The model under review builds one solid part; all positions refer to its coordinate system, in mm. Face numbers are marked on the shaded views. A direction names the side the tool comes from. Round coordinates to 2 decimals unless told otherwise and drop trailing zeros. Loops run counter-clockwise (first coordinate to the right, second up) from the corner with the lowest first, then second, coordinate; pieces in that order, holes last. Notation, with made-up numbers: (77, -7.5) -> (117, -7.5) arc R26 ccw to (117, 9.5) -> close; hole circle Ø3 at (21, 16.5). An arc over 180 degrees is marked (long way). Use CSV: the item, a comma, the result in double quotes. Start each with the question number.
```python
from build123d import *

# Parameters (mm, degrees)
SKETCH1_R               = 27.274244274
SKETCH1_R_2             = 12.5
BOSS_EXTRUDE1_DEPTH     = 2
SKETCH4_R               = 15
BOSS_EXTRUDE3_DEPTH     = 7
SKETCH5_R               = 6
SKETCH5_R_2             = 4.1
BOSS_EXTRUDE4_DEPTH     = 10
CUT_EXTRUDE1_DEPTH      = 43.997311561
CUT_EXTRUDE1_DEPTH_BACK = 43.997311561
SKETCH6_R               = 1.55
SKETCH7_R               = 7.5
CUT_EXTRUDE2_DEPTH      = 5
CUT_EXTRUDE3_DEPTH      = 43.151735491
CUT_EXTRUDE3_DEPTH_BACK = 43.151735491
SKETCH9_R               = 1.1


with BuildPart() as part:
    # Sketch1 → Boss-Extrude1 (new body)
    with BuildSketch(Plane(origin=(0, 0, 0), x_dir=(1, 0, 0), z_dir=(0, 1, 0))):
        with Locations(Location((0, 0, 0), (0, 0, 270))):
            Circle(SKETCH1_R)
        with Locations(Location((0, 0, 0), (0, 0, 270))):
            Circle(SKETCH1_R_2, mode=Mode.SUBTRACT)
    extrude(amount=BOSS_EXTRUDE1_DEPTH)

    # Sketch4 → Boss-Extrude3 (add)
    with BuildSketch(Plane(origin=(0, 2, 0), x_dir=(1, 0, 0), z_dir=(0, 1, 0))):
        with Locations(Location((0, 0, 0), (0, 0, 270))):
            Circle(SKETCH4_R)
    extrude(amount=BOSS_EXTRUDE3_DEPTH)

    # Sketch5 → Boss-Extrude4 (add)
    with BuildSketch(Plane(origin=(0, 9, 0), x_dir=(1, 0, 0), z_dir=(0, 1, 0))):
        with Locations(Location((0, 0, 0), (0, 0, 270))):
            Circle(SKETCH5_R)
        with Locations(Location((0, 0, 0), (0, 0, 270))):
            Circle(SKETCH5_R_2, mode=Mode.SUBTRACT)
    extrude(amount=BOSS_EXTRUDE4_DEPTH)

    # Sketch6 → Cut-Extrude1 (cut, two sides: drawn at the far end of the back side and taken through both)
    with BuildSketch(Plane(origin=(0, 0, 0), x_dir=(0, 0, -1), z_dir=(1, 0, 0)).offset(-CUT_EXTRUDE1_DEPTH_BACK)):
        with Locations((0, 15.818596456)):
            Circle(SKETCH6_R)
    extrude(amount=CUT_EXTRUDE1_DEPTH + CUT_EXTRUDE1_DEPTH_BACK, mode=Mode.SUBTRACT)

    # Sketch7 → Cut-Extrude2 (cut)
    with BuildSketch(Plane.XZ.offset(-2)):
        with Locations(Location((0, 0, 0), (0, 0, 270))):
            Circle(SKETCH7_R)
    extrude(amount=-CUT_EXTRUDE2_DEPTH, mode=Mode.SUBTRACT)

    # Sketch9 → Cut-Extrude3 (cut, two sides: drawn at the far end of the back side and taken through both)
    with BuildSketch(Plane(origin=(0, 2, 0), x_dir=(1, 0, 0), z_dir=(0, 1, 0)).offset(-CUT_EXTRUDE3_DEPTH_BACK)):
        with Locations(Location((0, 17, 0), (0, 0, 270))):
            Circle(SKETCH9_R)
        with Locations(Location((14.722431864, 8.5, 0), (0, 0, 270))):
            Circle(SKETCH9_R)
        with Locations(Location((14.722431864, -8.5, 0), (0, 0, 270))):
            Circle(SKETCH9_R)
        with Locations(Location((0, -17, 0), (0, 0, 270))):
            Circle(SKETCH9_R)
        with Locations(Location((-14.722431864, -8.5, 0), (0, 0, 270))):
            Circle(SKETCH9_R)
        with Locations(Location((-14.722431864, 8.5, 0), (0, 0, 270))):
            Circle(SKETCH9_R)
    extrude(amount=CUT_EXTRUDE3_DEPTH + CUT_EXTRUDE3_DEPTH_BACK, mode=Mode.SUBTRACT)


solid = part.part
```
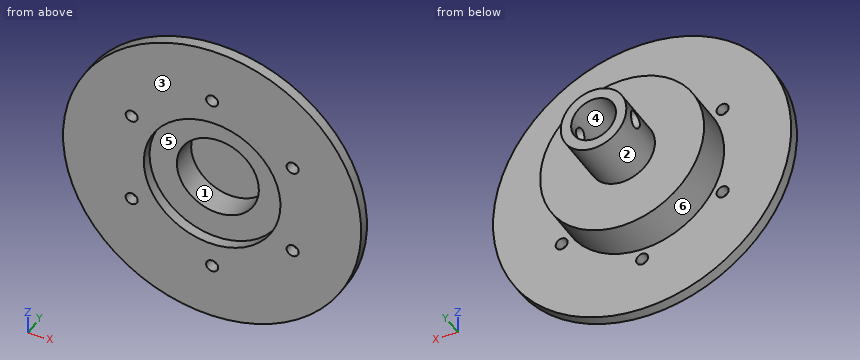
1. Clearance check with flat-ended pins moving along their axes: P1, Ø5, axis at y = 10.5, z = 2.5, coming from the -X side; P2, Ø6.5, axis at x = 0, z = 0, coming from the -Y side; P3, Ø8, axis at x = 3.5, z = 3, coming from the -Y side; P4, Ø1.9, axis at y = 15.82, z = 0, coming from the -X side. State where each tip first meets the part, or that it passes through.
2. For the marked faces 1 and 2, list the 3-axis set-ups (+Z, -Z, +X, -X, +Y, -Y) from which the entire face can be reached by the end or side of a thin tool; tool diameter is ignored.
3. Take a section at D-D, the plane y = 10. Give the boundary of the cut face in (x, z).
4. For line 1 along X through (y, z) = (1.5, 8.5); line 2 along Y through (x, z) = (5.25, 0); line 3 along Y through (x, z) = (-23, -12), list the stretches that pass through material, from the lowest coordinate up. Write a range as from..to.
5. Take a section at C-C, the plane z = -17. Give the boundary of the cut face in (x, y).
6. The part is to be moulded in two halves that separate along Z. For the marked faces 3, 4, 5 and 6, say which applies: pulls with the +Z half, pulls with the -Z half, needs draft (parallel to the pull), parting line crosses it, or undercut.
7. Take a section at A-A, the plane x = 0. Count the separate pieces of the cut face and the enclosed holes in it, then the cut area to 3 significant figures.
Results:
1,P1,"x = -14.99"
1,P2,"y = 7"
1,P3,"y = 2"
1,P4,"through"
2,face 1,"-Y"
2,face 2,"+Y"
3,outline,"circle Ø12 at (0, 0); hole circle Ø8.2 at (0, 0)"
4,line 1,"-25.92..-15.82, -13.62..-9.17, 9.17..13.62, 15.82..25.92"
4,line 2,"7..14.27, 17.37..19"
4,line 3,"0..2"
5,outline,"(-21.33, 0) -> (-1.1, 0) -> (-1.1, 2) -> (-21.33, 2) -> close; (1.1, 0) -> (21.33, 0) -> (21.33, 2) -> (1.1, 2) -> close"
6,face 3,"needs draft"
6,face 4,"undercut"
6,face 5,"undercut"
6,face 6,"parting line crosses it"
7,separate pieces,"3"
7,enclosed holes,"0"
7,area,"223 mm²"
